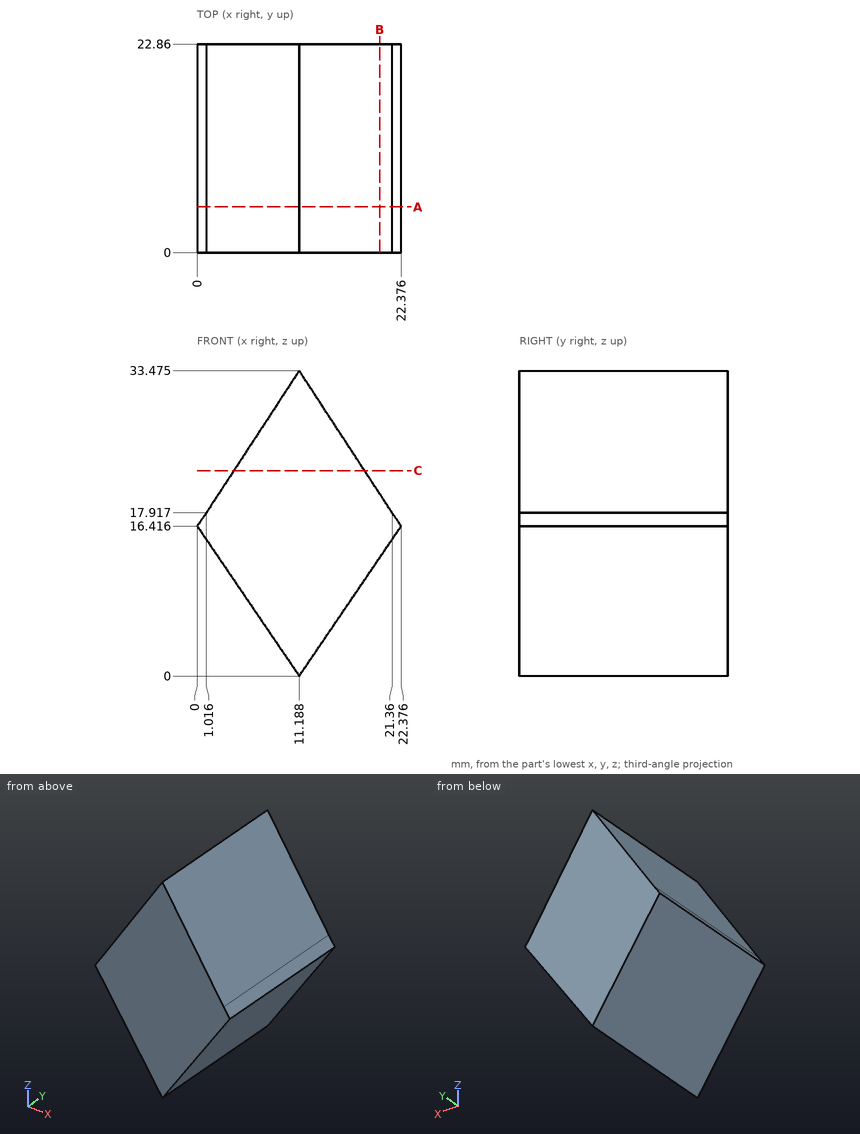
Geometry: see drawing. Coordinates: mm, zero at the bounding-box minimum. Give positions to 0.01 mm unless a question says otherwise; leave off trailing zeros. Loops run counter-clockwise (first coordinate to the right, second up) from the corner with the lowest first, then second, coordinate; pieces in that order, holes last. Notation, with made-up numbers: (45.25, 26.5) - (79.25, 26.5) arc R16 cw to (79.25, 39.5) - close; hole circle Ø10 at (81.5, 39). An arc over 180 degrees is marked (long way). One line per question, with ' | ' between items. Start each with the question number.
(1) Section query A-A on y = 5. Return loops of the section in (x, z) (1 decimal), then the cut area to 3 significant figures.
(2) Section query B-B on x = 20. Return loops of the section in (y, z), then the cut area to 3 significant figures.
(3) Ray query, line 1 (X direction, y = 22, z = 6); line 2 (Z direction, x = 5.5, y = 2.5) (1 decimal); line 3 (Z direction, x = 20.25, y = 1.5) (1 decimal). Return the intervals inside material, ascending. Write a range as from..to.
(4) Contact query for flat-ended pins moving along their axis: pin 1 (1 mm diameter, centred on y = 13, z = 18, fed in from -X); pin 2 (2 mm diameter, centred on y = 2.5, z = 15, fed in from -X) (1 decimal); pin 3 (5 mm diameter, centred on x = 19.5, y = 7.5, fed in from +Z) (1 decimal). Output: stop coordinate, or through.
(5) Section query C-C on z = 22.5. Return loops of the section in (x, y).
The answers:
1) outline: (0, 16.4) - (11.2, 0) - (22.4, 16.4) - (21.4, 17.9) - (11.2, 33.5) - (1, 17.9) - close | area: 374 mm2
2) outline: (0, 12.93) - (22.86, 12.93) - (22.86, 20) - (0, 20) - close | area: 162 mm2
3) line 1: 7.1..15.28 | line 2: 8.3..24.8 | line 3: 13.3..19.6
4) pin 1: x = 0.73 | pin 2: x = 0.3 | pin 3: z = 24.6
5) outline: (4.01, 0) - (18.36, 0) - (18.36, 22.86) - (4.01, 22.86) - close
